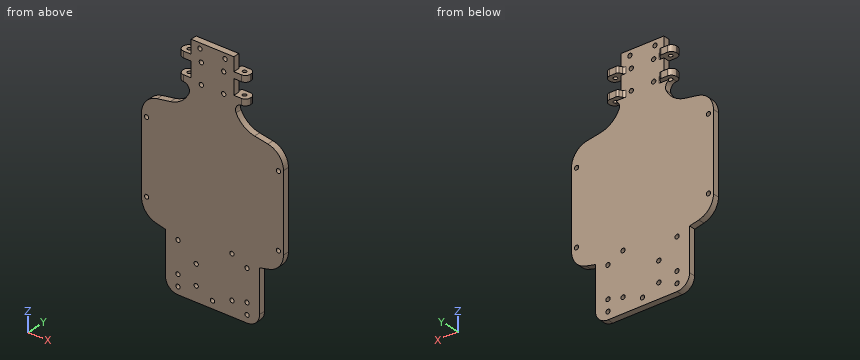
```python
from build123d import *

# Parameters (mm, degrees)
BOSS_EXTRU_1_DEPTH      = 5
CONG_1_R                = 20
CONG_2_R                = 5
BOSS_EXTRU_2_DEPTH      = 5
CONG_4_R                = 2
CONG_5_R                = 4
ESQUISSE3_R             = 1.5
ENL_V_MAT_EXTRU_2_DEPTH = 25
ESQUISSE4_R             = 1.7
ENL_V_MAT_EXTRU_3_DEPTH = 25
ESQUISSE5_R             = 1.7
ENL_V_MAT_EXTRU_4_DEPTH = 10
ESQUISSE6_R             = 1.7
ENL_V_MAT_EXTRU_5_DEPTH = 10
CONG_6_R                = 10


with BuildPart() as part:
    # Esquisse1 → Boss.-Extru.1 (new body)
    with BuildSketch(Plane(origin=(0, 0, 0), x_dir=(1, 0, 0), z_dir=(0, 1, 0))):
        with BuildLine():
            Line((-37.5, 95), (37.5, 95))
            Line((37.5, 95), (37.5, 51))
            Line((37.5, 51), (44.874265815, 49.29751659))
            ThreePointArc((44.874265815, 49.29751659), (53.239122353, 44.019685168), (56.5, 34.681965619))
            Line((56.5, 34.681965619), (56.5, -26.800001164))
            ThreePointArc((56.5, -26.800001164), (52.990666647, -36.441815309), (44.104722665, -41.572117459))
            Line((44.104722665, -41.572117459), (17, -46.351411369))
            Line((17, -46.351411369), (17, -61.9))
            Line((17, -61.9), (27, -61.9))
            Line((27, -61.9), (27, -66.9))
            Line((27, -66.9), (17, -66.9))
            Line((17, -66.9), (17, -79.1))
            Line((17, -79.1), (27, -79.1))
            Line((27, -79.1), (27, -84.1))
            Line((27, -84.1), (17, -84.1))
            Line((17, -84.1), (17, -95))
            Line((17, -95), (-17, -95))
            Line((-17, -95), (-17, -84.1))
            Line((-17, -84.1), (-27, -84.1))
            Line((-27, -84.1), (-27, -79.1))
            Line((-27, -79.1), (-17, -79.1))
            Line((-17, -79.1), (-17, -66.9))
            Line((-17, -66.9), (-27, -66.9))
            Line((-27, -66.9), (-27, -61.9))
            Line((-27, -61.9), (-17, -61.9))
            Line((-17, -61.9), (-17, -46.351411369))
            Line((-17, -46.351411369), (-44.104722665, -41.572117459))
            ThreePointArc((-44.104722665, -41.572117459), (-52.990666647, -36.441815309), (-56.5, -26.800001164))
            Line((-56.5, -26.800001164), (-56.5, 34.681965619))
            ThreePointArc((-56.5, 34.681965619), (-53.239122353, 44.019685168), (-44.874265815, 49.29751659))
            Line((-44.874265815, 49.29751659), (-37.5, 51))
            Line((-37.5, 51), (-37.5, 95))
        make_face()
    extrude(amount=BOSS_EXTRU_1_DEPTH)

    # Congé1
    # the kernel refuses this fillet: 20 mm, written as the material it adds along each edge
    with BuildSketch(Plane(origin=(17, 0, 46.351411369), x_dir=(0.9848077530122094, 0, -0.1736481776669235), z_dir=(0, 1, 0))) as cong_1_piece_1:
        with BuildLine():
            CenterArc((16.742910017, -20), CONG_1_R, 90, 76.444834731)
            Line((-2.699984081, -15.312370632), (-3.088841963, -15.218618044))
            ThreePointArc((-3.088841963, -15.218618044), (-1.743915142, -7.586726045), (-0.393923101, 0.069459271))
            Line((-0.393923101, 0.069459271), (0, 0.4))
            Line((0, 0.4), (16.742910017, 0.4))
            Line((16.742910017, 0.4), (16.742910017, 0))
        make_face()
    extrude(amount=5)
    with BuildSketch(Plane(origin=(-17, 0, 46.351411369), x_dir=(0, 0, 1), z_dir=(0, 1, 0))) as cong_1_piece_2:
        with BuildLine():
            CenterArc((16.788779247, -19.961511146), CONG_1_R, 93.555165269, 76.444834731)
            Line((-2.907375813, -16.488547593), (-3.301298915, -16.419088322))
            Line((-3.301298915, -16.419088322), (-0.393923101, 0.069459271))
            Line((-0.393923101, 0.069459271), (0, 0.4))
            ThreePointArc((0, 0.4), (7.774294315, 0.4), (15.523784818, 0.399230223))
            Line((15.523784818, 0.399230223), (15.548588631, 0))
        make_face()
    extrude(amount=5)

    # Congé2
    cong_2_edges = [part.edges().sort_by_distance(p)[0] for p in [
        (-17, 2.5, 61.9),
        (17, 2.5, 61.9),
    ]]
    fillet(cong_2_edges, radius=CONG_2_R)

    # Esquisse2 → Boss.-Extru.2 (add)
    with BuildSketch(Plane.XY.offset(84.1)):
        Polygon((-27, 5), (-27, 8.904402326), (-16.833134842, 8.904402326), (-14.427579086, 5), (-14.427579086, 0), (-27, 0), align=None)
        Polygon((16.833134842, 8.904402326), (14.427579086, 5), (14.427579086, 0), (27, 0), (27, 5), (27, 8.904402326), align=None)
    boss_extru_2 = extrude(amount=-BOSS_EXTRU_2_DEPTH)

    # Symétrie1: Boss.-Extru.2 across plane
    add(boss_extru_2.mirror(Plane.XY.offset(73)))

    # Congé4
    cong_4_edges = [part.edges().sort_by_distance(p)[0] for p in [
        (16.833134842, 8.904402326, 81.6),
        (14.427579086, 5, 81.6),
        (-16.833134842, 8.904402326, 81.6),
        (-14.427579086, 5, 81.6),
        (16.833134842, 8.904402326, 64.4),
        (14.427579086, 5, 64.4),
        (-14.427579086, 5, 64.4),
        (-16.833134842, 8.904402326, 64.4),
    ]]
    fillet(cong_4_edges, radius=CONG_4_R)

    # Congé5
    cong_5_edges = [part.edges().sort_by_distance(p)[0] for p in [
        (27, 8.904402326, 81.6),
        (-27, 8.904402326, 81.6),
        (27, 8.904402326, 64.4),
        (-27, 8.904402326, 64.4),
        (-27, 0, 64.4),
        (-27, 0, 81.6),
        (27, 0, 81.6),
        (27, 0, 64.4),
    ]]
    fillet(cong_5_edges, radius=CONG_5_R)

    # Esquisse3 → Enlèv. mat.-Extru.2 (cut)
    with BuildSketch(Plane.XY.offset(84.1)):
        with Locations((-22, 4.452201163)):
            Circle(ESQUISSE3_R)
        with Locations(Location((22, 4.452201163, 0), (0, 0, 331.733302731))):
            Circle(ESQUISSE3_R)
    extrude(amount=-ENL_V_MAT_EXTRU_2_DEPTH, mode=Mode.SUBTRACT)

    # Esquisse4 → Enlèv. mat.-Extru.3 (cut)
    with BuildSketch(Plane(origin=(0, 5, 0), x_dir=(1, 0, 0), z_dir=(0, 1, 0))):
        with Locations(Location((-10, -90.8, 0), (0, 0, 270))):
            Circle(ESQUISSE4_R)
        with Locations(Location((10, -90.8, 0), (0, 0, 270))):
            Circle(ESQUISSE4_R)
        with Locations(Location((8.90673672, -64.828011588, 0), (0, 0, 270))):
            Circle(ESQUISSE4_R)
        with Locations(Location((8.90673672, -81.171988412, 0), (0, 0, 270))):
            Circle(ESQUISSE4_R)
        with Locations(Location((-8.90673672, -81.171988412, 0), (0, 0, 270))):
            Circle(ESQUISSE4_R)
        with Locations(Location((-8.90673672, -64.828011588, 0), (0, 0, 270))):
            Circle(ESQUISSE4_R)
    extrude(amount=-ENL_V_MAT_EXTRU_3_DEPTH, mode=Mode.SUBTRACT)

    # Esquisse5 → Enlèv. mat.-Extru.4 (cut)
    with BuildSketch(Plane(origin=(0, 5, 0), x_dir=(1, 0, 0), z_dir=(0, 1, 0))):
        with Locations(Location((15.5, 83, 0), (0, 0, 270))):
            Circle(ESQUISSE5_R)
        with Locations(Location((15.5, 49, 0), (0, 0, 270))):
            Circle(ESQUISSE5_R)
        with Locations(Location((-13, 83, 0), (0, 0, 270))):
            Circle(ESQUISSE5_R)
        with Locations(Location((-13, 67, 0), (0, 0, 270))):
            Circle(ESQUISSE5_R)
        with Locations(Location((27.5, 80, 0), (0, 0, 270))):
            Circle(ESQUISSE5_R)
        with Locations(Location((27.5, 55, 0), (0, 0, 270))):
            Circle(ESQUISSE5_R)
        with Locations(Location((27.5, 89, 0), (0, 0, 270))):
            Circle(ESQUISSE5_R)
        with Locations(Location((-27.5, 89, 0), (0, 0, 270))):
            Circle(ESQUISSE5_R)
        with Locations(Location((-27.5, 80, 0), (0, 0, 270))):
            Circle(ESQUISSE5_R)
        with Locations(Location((-27.5, 55, 0), (0, 0, 270))):
            Circle(ESQUISSE5_R)
        with Locations(Location((0, 89, 0), (0, 0, 270))):
            Circle(ESQUISSE5_R)
    extrude(amount=-ENL_V_MAT_EXTRU_4_DEPTH, mode=Mode.SUBTRACT)

    # Esquisse6 → Enlèv. mat.-Extru.5 (cut)
    with BuildSketch(Plane(origin=(0, 5, 0), x_dir=(1, 0, 0), z_dir=(0, 1, 0))):
        with Locations(Location((-52.484739006, 32.940982227, 0), (0, 0, 270))):
            Circle(ESQUISSE6_R)
        with Locations(Location((-52.484739006, -25.059017773, 0), (0, 0, 270))):
            Circle(ESQUISSE6_R)
        with Locations(Location((52.484739006, -25.059017773, 0), (0, 0, 90))):
            Circle(ESQUISSE6_R)
        with Locations(Location((52.484739006, 32.940982227, 0), (0, 0, 90))):
            Circle(ESQUISSE6_R)
    extrude(amount=-ENL_V_MAT_EXTRU_5_DEPTH, mode=Mode.SUBTRACT)

    # Congé6
    cong_6_edges = [part.edges().sort_by_distance(p)[0] for p in [
        (37.5, 2.5, -95),
        (-37.5, 2.5, -95),
    ]]
    fillet(cong_6_edges, radius=CONG_6_R)


solid = part.part
```
CAD build for the part. Positions are in the model's coordinates, mm. Give positions to 0.01 mm unless a question says otherwise; leave off trailing zeros. Order: outer loops, then holes, each group sorted by start corner. A loop starts at its lowest first (then second) coordinate and runs counter-clockwise, first axis right, second up.
(1) Drill centre lines: L1, parallel to X at y = 3.8, z = -83; L2, parallel to Z at x = 28, y = 1.5; L3, parallel to Y at x = 37.5, z = -45. Where is each one in solid material? Low to high.
(2) Saw through at B-B, the plane z = 1.5. Give the cut face in (x, y), then the cut area to 3 significant figures.
(3) Saw through at A-A, the plane x = -5. Give the cut face in (y, z).
(4) Flat gauge pins, fed straight in: pin 1 (5 mm diameter, centred on x = -15, z = 11, fed in from +Y); pin 2 (1 mm diameter, centred on y = 4.5, z = 65.5, fed in from +X); pin 3 (1.5 mm diameter, centred on y = 1.5, z = -73, fed in from -X). Where does each tip first touch, or does it go through?
Results found:
1. L1: x = -37.5 to -14.7, -11.3 to 13.8, 17.2 to 37.5
1. L2: z = -94.99 to -90.62, -87.38 to -81.62, -78.38 to -56.62, -53.38 to 45.26
1. L3: y = 0 to 5
2. outline: (-56.5, 0) - (56.5, 0) - (56.5, 5) - (-56.5, 5) - close
2. area: 565 mm2
3. outline: (0, -95) - (5, -95) - (5, 95) - (0, 95) - close
4. pin 1: stops at y = 5
4. pin 2: stops at x = 27
4. pin 3: stops at x = -37.5
